```python
from build123d import *

# Parameters (mm, degrees)
SKETCH1_W           = 160
SKETCH1_H           = 120
BOSS_EXTRUDE1_DEPTH = 3
SKETCH2_R           = 3
BOSS_EXTRUDE2_DEPTH = 28
SKETCH3_W           = 56
SKETCH3_H           = 86
CUT_EXTRUDE1_DEPTH  = 1.5
SKETCH5_W           = 52
SKETCH5_H           = 66
CUT_EXTRUDE2_DEPTH  = 1.5


with BuildPart() as part:
    # Sketch1 → Boss-Extrude1 (new body)
    with BuildSketch(Plane(origin=(0, 0, 0), x_dir=(1, 0, 0), z_dir=(0, 1, 0))):
        Rectangle(SKETCH1_W, SKETCH1_H)
    extrude(amount=BOSS_EXTRUDE1_DEPTH)

    # Sketch2 → Boss-Extrude2 (add)
    with BuildSketch(Plane(origin=(0, 3, 0), x_dir=(1, 0, 0), z_dir=(0, 1, 0))):
        with Locations(Location((-70, 50, 0), (0, 0, 90))):
            Circle(SKETCH2_R)
        with Locations(Location((0, 50, 0), (0, 0, 90))):
            Circle(SKETCH2_R)
        with Locations(Location((70, 50, 0), (0, 0, 90))):
            Circle(SKETCH2_R)
        with Locations(Location((-70, 0, 0), (0, 0, 90))):
            Circle(SKETCH2_R)
        with Locations(Location((70, 0, 0), (0, 0, 90))):
            Circle(SKETCH2_R)
        with Locations(Location((-70, -50, 0), (0, 0, 90))):
            Circle(SKETCH2_R)
        with Locations(Location((0, -50, 0), (0, 0, 90))):
            Circle(SKETCH2_R)
        with Locations(Location((70, -50, 0), (0, 0, 90))):
            Circle(SKETCH2_R)
    extrude(amount=BOSS_EXTRUDE2_DEPTH)

    # Sketch3 → Cut-Extrude1 (cut)
    with BuildSketch(Plane(origin=(0, 3, 0), x_dir=(1, 0, 0), z_dir=(0, 1, 0))):
        with Locations((-35, 0)):
            Rectangle(SKETCH3_W, SKETCH3_H)
    extrude(amount=-CUT_EXTRUDE1_DEPTH, mode=Mode.SUBTRACT)

    # Sketch5 → Cut-Extrude2 (cut)
    with BuildSketch(Plane(origin=(0, 3, 0), x_dir=(1, 0, 0), z_dir=(0, 1, 0))):
        with Locations((38, 0)):
            Rectangle(SKETCH5_W, SKETCH5_H)
    extrude(amount=-CUT_EXTRUDE2_DEPTH, mode=Mode.SUBTRACT)


solid = part.part
```
Build history of the part. All positions in model axes, mm. A direction names the side the tool comes from. Round coordinates to 2 decimals unless told otherwise and drop trailing zeros. Loops run counter-clockwise (first coordinate to the right, second up) from the corner with the lowest first, then second, coordinate; pieces in that order, holes last.
Item 1: Saw through at C-C (z = 50). List the corners of the cut face in (x, y), then the cut area to 3 significant figures.
Item 2: Drill centre lines: line 1 along Z through (x, y) = (-67.5, 24.5); line 2 along X through (y, z) = (24, -52.5); line 3 along X through (y, z) = (25, -49). Where is each one in solid material? Low to high.
Item 3: Saw through at A-A (y = 20.5). List the corners of the cut face in (x, z), then the cut area to 3 significant figures.
Item 4: Which spindle directions (+Z, -Z, +X, -X, +Y, -Y) get a long thin tool onto all of the face, cutting with end or side? Do faces 1 (the face through (0, 17, 53)), 2 (the face through (-1, 0, -1)). Say none if no direction does.
Item 5: Saw through at B-B (x = 29). List the corners of the cut face in (y, z), then the cut area to 3 significant figures.
Item 6: Saw through at D-D (z = 0). List the corners of the cut face in (x, y), then the cut area to 3 significant figures.
Item 7: Two-plate mould, pull along Z, no slides. Class faces 3 (the face through (38, 1.5, 0)), 4 (the face through (-70, 31, -50)): released by +Z, released by -Z, zero draft, split by the parting line, or undercut.
Item 8: Pin check, flat tips, straight feed: P1, Ø10, axis at y = 7, z = -6.5, coming from the +X side; P2, Ø15.5, axis at x = 35.5, z = 16, coming from the +Y side; P3, Ø3, axis at x = 27, z = 32.5, coming from the +Y side; P4, Ø10, axis at y = 10.5, z = 45.5, coming from the +X side. Stop position of each tip, or through.
Worked answers:
1. outline: (-80, 0) - (80, 0) - (80, 3) - (73, 3) - (73, 31) - (67, 31) - (67, 3) - (3, 3) - (3, 31) - (-3, 31) - (-3, 3) - (-67, 3) - (-67, 31) - (-73, 31) - (-73, 3) - (-80, 3) - close
1. area: 984 mm2
2. line 1: z = -51.66 to -48.34, -1.66 to 1.66, 48.34 to 51.66
2. line 2: x = -71.66 to -68.34, -1.66 to 1.66, 68.34 to 71.66
2. line 3: x = -72.83 to -67.17, -2.83 to 2.83, 67.17 to 72.83
3. outline: circle Ø6 at (-70, -50); circle Ø6 at (-70, 0); circle Ø6 at (-70, 50); circle Ø6 at (0, -50); circle Ø6 at (0, 50); circle Ø6 at (70, -50); circle Ø6 at (70, 0); circle Ø6 at (70, 50)
3. area: 226 mm2
4. face 1: +Y
4. face 2: +Z, -Z, +X, -X, -Y
5. outline: (0, -60) - (3, -60) - (3, -33) - (1.5, -33) - (1.5, 33) - (3, 33) - (3, 60) - (0, 60) - close
5. area: 261 mm2
6. outline: (-80, 0) - (80, 0) - (80, 3) - (73, 3) - (73, 31) - (67, 31) - (67, 3) - (64, 3) - (64, 1.5) - (12, 1.5) - (12, 3) - (-7, 3) - (-7, 1.5) - (-63, 1.5) - (-63, 3) - (-67, 3) - (-67, 31) - (-73, 31) - (-73, 3) - (-80, 3) - close
6. area: 654 mm2
7. face 3: undercut
7. face 4: zero draft
8. P1: stops at x = 80
8. P2: stops at y = 1.5
8. P3: stops at y = 3
8. P4: stops at x = 73
